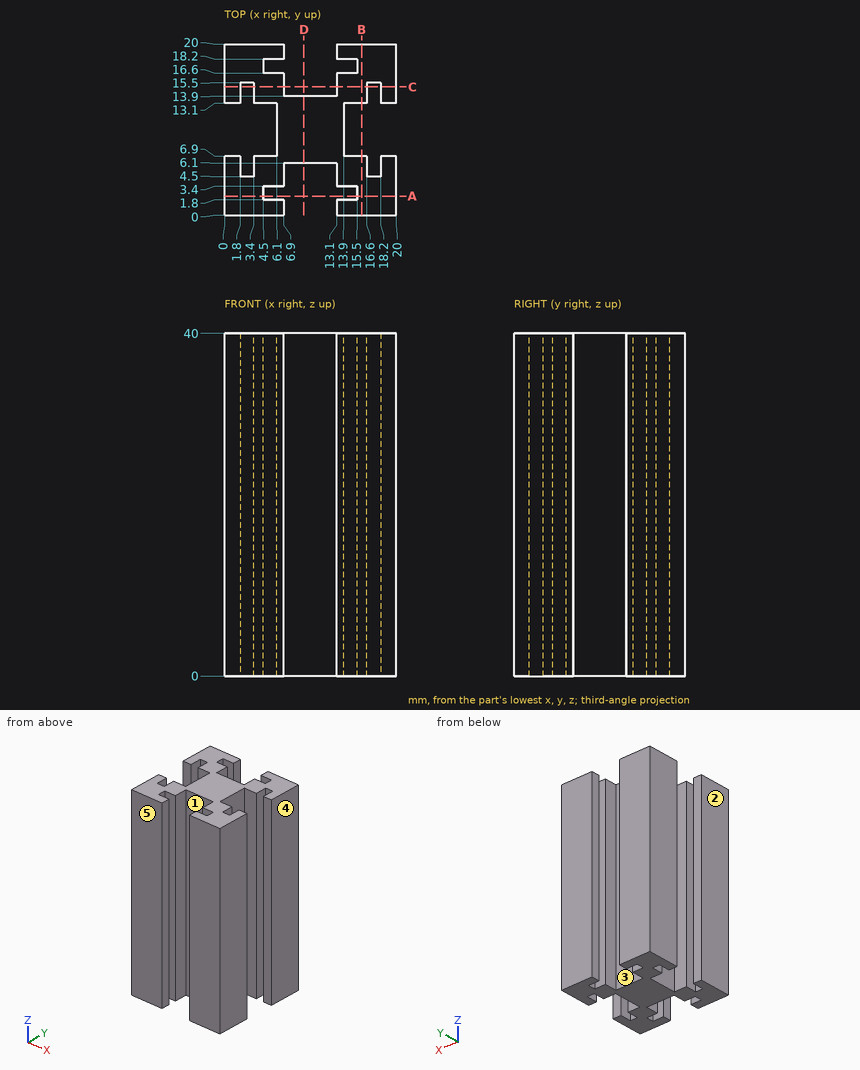
Could you check a few things on this drawing? It's one solid part, dimensions in mm from its lowest x, y, z. A direction names the side the tool comes from. Coordinates: 2 decimals unless noted, no trailing zeros. Write each loop counter-clockwise with the first axis right and the second up, starting at its lowest first coordinate (ties: lowest second). Pieces come first, ordered by that corner, then holes. Notation, with made-up numbers: M 48,14.25 L 76,14.25 A31 cw 76,38.25 Z; hole C 66,14.25 d3. An arc over 180 degrees is marked long. Answer as CSV lines item,"result". Start each with the question number.
Q1. Suppose I cut it at D-D, the plane x = 9.25. List the corners of the cut face in (y, z) for me.
Q2. Suppose I cut it at B-B, the plane x = 16. List the corners of the cut face in (y, z) for me, then the cut area to 3 significant figures.
Q3. I need wall thicknesses on probe 1 along X at (y, z) = (14, 10.5); probe 2 along Y at (x, z) = (6.75, 20.5); probe 3 along X at (y, z) = (17.75, 32.5). Which ranges of each line are inside material? Lowest first, please. Write a range as [from, to].
Q4. Will this pin go through, and if not, where does the flat tip stop? pin 1 Ø5 at (y, z) = (10, 25) entering from -X.
Q5. If we mould it in two halves opening along X, with no side actions, what happens to the marked faces 3, 4 and 5? For each: pulls with the +X half, pulls with the -X half, needs draft (parallel to the pull), parting line crosses it, or undercut.
Q6. Suppose I cut it at C-C, the plane y = 15. List the corners of the cut face in (x, z) for me.
Q7. For the marked faces 1 and 2, which set-ups out of +Z, -Z, +X, -X, +Y, -Y let a thin tool reach every point of the face, with its end or its side?
Q8. Suppose I cut it at A-A, the plane y = 2.25. List the corners of the cut face in (x, z) for me, then the cut area to 3 significant figures.
Entries:
1,outline,"M 6.1,0 L 13.9,0 L 13.9,40 L 6.1,40 Z"
2,outline,"M 0,0 L 6.9,0 L 6.9,40 L 0,40 Z; M 13.1,0 L 20,0 L 20,40 L 13.1,40 Z"
2,area,"552 mm²"
3,probe 1,"x = [0, 1.8], [3.4, 6.9], [13.1, 16.6], [18.2, 20]"
3,probe 2,"y = [0, 1.8], [3.4, 16.6], [18.2, 20]"
3,probe 3,"x = [0, 4.5], [15.5, 20]"
4,pin 1,"stops at x = 6.1"
5,face 3,"undercut"
5,face 4,"pulls with the +X half"
5,face 5,"needs draft"
6,outline,"M 0,0 L 1.8,0 L 1.8,40 L 0,40 Z; M 3.4,0 L 6.9,0 L 6.9,40 L 3.4,40 Z; M 13.1,0 L 16.6,0 L 16.6,40 L 13.1,40 Z; M 18.2,0 L 20,0 L 20,40 L 18.2,40 Z"
7,face 1,"+Z, -Z, -Y"
7,face 2,"+Z, -Z, -X, +Y, -Y"
8,outline,"M 0,0 L 4.5,0 L 4.5,40 L 0,40 Z; M 15.5,0 L 20,0 L 20,40 L 15.5,40 Z"
8,area,"360 mm²"
